Geometry check sheet. Reference: the model listing, model coordinates, mm. Round coordinates to 2 decimals unless told otherwise and drop trailing zeros. Write each loop counter-clockwise with the first axis right and the second up, starting at its lowest first coordinate (ties: lowest second). Pieces come first, ordered by that corner, then holes. Notation, with made-up numbers: (27.25, 37.25) - (53.25, 37.25) arc R34 ccw to (53.25, 73.25) - close; hole circle Ø11 at (47, 35.5). An arc over 180 degrees is marked (long way). Return JSON: item names as keys, results as strings.
```python
from build123d import *

# Parameters (mm, degrees)
SKETCH1_W           = 466
SKETCH1_H           = 126.5
BOSS_EXTRUDE1_DEPTH = 6
SKETCH2_W           = 514
SKETCH2_H           = 174.5
SKETCH2_W_2         = 68.285714286
SKETCH2_H_2         = 6
SKETCH2_W_3         = 68.285714285
SKETCH2_W_4         = 73.428571428
SKETCH2_W_5         = 6
SKETCH2_H_3         = 25.3
SKETCH2_H_4         = 37.3
BOSS_EXTRUDE2_DEPTH = 6


with BuildPart() as part:
    # Sketch1 → Boss-Extrude1 (new body)
    with BuildSketch(Plane(origin=(0, 0, 0), x_dir=(1, 0, 0), z_dir=(0, 1, 0))):
        Rectangle(SKETCH1_W, SKETCH1_H)
    extrude(amount=BOSS_EXTRUDE1_DEPTH)

    # Sketch2 → Boss-Extrude2 (add)
    with BuildSketch(Plane(origin=(0, 6, 0), x_dir=(1, 0, 0), z_dir=(0, 1, 0))):
        Rectangle(SKETCH2_W, SKETCH2_H)
        Polygon((170.714285714, 69.25), (102.428571429, 69.25), (34.142857143, 69.25), (-34.142857143, 69.25), (-102.428571429, 69.25), (-170.714285714, 69.25), (-239, 69.25), (-239, 63.25), (-239, 37.95), (-239, 12.65), (-239, -12.65), (-239, -37.95), (-239, -63.25), (-239, -69.25), (239, -69.25), (239, 69.25), align=None, mode=Mode.SUBTRACT)
        with Locations((0, 66.25)):
            Rectangle(SKETCH2_W_2, SKETCH2_H_2)
        with Locations((-136.571428572, 66.25)):
            Rectangle(SKETCH2_W_3, SKETCH2_H_2)
        with Locations((136.571428572, 66.25)):
            Rectangle(SKETCH2_W_3, SKETCH2_H_2)
        with Locations((-146.857142857, 90.25)):
            Rectangle(SKETCH2_W_4, SKETCH2_H_2)
        with Locations((0, 90.25)):
            Rectangle(SKETCH2_W_4, SKETCH2_H_2)
        with Locations((146.857142857, 90.25)):
            Rectangle(SKETCH2_W_4, SKETCH2_H_2)
        with Locations((-236, 50.6)):
            Rectangle(SKETCH2_W_5, SKETCH2_H_3)
        Polygon((-263, 55.95), (-257, 55.95), (-257, 87.25), (-257, 93.25), (-263, 93.25), align=None)
        with Locations((-236, 0)):
            Rectangle(SKETCH2_W_5, SKETCH2_H_3)
        with Locations((-260, 0)):
            Rectangle(SKETCH2_W_5, SKETCH2_H_4)
        with Locations((-236, -50.6)):
            Rectangle(SKETCH2_W_5, SKETCH2_H_3)
        Polygon((-257, -93.25), (-257, -87.25), (-257, -55.95), (-263, -55.95), (-263, -93.25), align=None)
    boss_extrude2 = extrude(amount=-BOSS_EXTRUDE2_DEPTH)

    # Mirror2: Boss-Extrude2 across plane
    add(boss_extrude2.mirror(Plane.XY))

    # Mirror3: Boss-Extrude2 across plane
    add(boss_extrude2.mirror(Plane(origin=(0, 0, 0), x_dir=(0, 0, 1), z_dir=(1, 0, 0))))


solid = part.part
```
(1) Section check A-A, the plane x = -92. Enter the section's corners in (y, z).
Response values:
{"outline": "(0, -87.25) - (6, -87.25) - (6, -69.25) - (0, -69.25) - close; (0, -63.25) - (6, -63.25) - (6, 63.25) - (0, 63.25) - close; (0, 69.25) - (6, 69.25) - (6, 87.25) - (0, 87.25) - close"}
(2) Section check C-C, the plane y = 3.3. Give the number of separate pieces and of enclosed holes in the cut face, plus the area to 3 significant figures.
Response values:
{"separate pieces": "1", "enclosed holes": "12", "area": "89,800 mm^2"}
(3) Gauge pin test, flat ends, axial feed: pin 1 (1.8 mm diameter, centred on x = -211.5, y = 4, fed in from +Z); pin 2 (1.8 mm diameter, centred on y = 4.5, z = -31, fed in from +X); pin 3 (2 mm diameter, centred on x = -47.5, y = 2, fed in from -Z). Record the tip position at first contact, or that the pin passes through.
Response values:
{"pin 1": "stops at z = 87.25", "pin 2": "stops at x = 257", "pin 3": "stops at z = -87.25"}
(4) Section check D-D, the plane z = -45.5. Enter the section's corners in (x, y), plus the area to 3 significant figures.
Response values:
{"outline": "(-257, 0) - (257, 0) - (257, 6) - (-257, 6) - close", "area": "3,080 mm^2"}
(5) Material ranges on line 1 along X through (y, z) = (1.65, -13.5); line 2 along Z through (x, y) = (-45.5, 2.55); line 3 along X through (y, z) = (1.55, 34), recorded low to high. Write a range as [from, to].
Response values:
{"line 1": "x = [-263, -239], [-233, 233], [239, 263]", "line 2": "z = [-87.25, -69.25], [-63.25, 63.25], [69.25, 87.25]", "line 3": "x = [-257, -239], [-233, 233], [239, 257]"}
(6) Section check B-B, the plane z = -25. Enter the section's corners in (x, y), plus the area to 3 significant figures.
Response values:
{"outline": "(-257, 0) - (-239, 0) - (-239, 6) - (-257, 6) - close; (-233, 0) - (233, 0) - (233, 6) - (-233, 6) - close; (239, 0) - (257, 0) - (257, 6) - (239, 6) - close", "area": "3,010 mm^2"}
